from build123d import *

# Parameters (mm, degrees)
BASE_FLANGE1_DEPTH = 280
SKETCH2_W          = 105.722877612
SKETCH2_H          = 35.527417617
CUT_EXTRUDE1_DEPTH = 10
SKETCH3_R          = 38
CUT_EXTRUDE2_DEPTH = 500


# Sheet-metal steps are written as plain solids
with BuildPart() as part:
    # Sketch1 → Base-Flange1 (new body)
    with BuildSketch(Plane(origin=(0, 0, 0), x_dir=(-1, 0, 0), z_dir=(0, 0, 1))):
        with BuildLine():
            Line((223.448991217, -255.847131966), (223.448991217, 313.416268034))
            ThreePointArc((223.448991217, 313.416268034), (223.233246072, 313.937122889), (222.712391217, 314.152868034))
            Line((222.712391217, 314.152868034), (-112.814408783, 314.152868034))
            ThreePointArc((-112.814408783, 314.152868034), (-113.335263638, 313.937122889), (-113.551008783, 313.416268034))
            Line((-113.551008783, 313.416268034), (-113.551008783, -255.847131966))
            Line((-113.551008783, -255.847131966), (-115.051008783, -255.847131966))
            Line((-115.051008783, -255.847131966), (-115.051008783, 313.416268034))
            ThreePointArc((-115.051008783, 313.416268034), (-114.39592381, 314.997783061), (-112.814408783, 315.652868034))
            Line((-112.814408783, 315.652868034), (222.712391217, 315.652868034))
            ThreePointArc((222.712391217, 315.652868034), (224.293906243, 314.997783061), (224.948991217, 313.416268034))
            Line((224.948991217, 313.416268034), (224.948991217, -255.847131966))
            Line((224.948991217, -255.847131966), (223.448991217, -255.847131966))
        make_face()
    extrude(amount=BASE_FLANGE1_DEPTH)

    # Sketch2 → Cut-Extrude1 (cut)
    with BuildSketch(Plane.ZY.offset(224.948991217)):
        with Locations((233.67908011, -135.779600883)):
            Rectangle(SKETCH2_W, SKETCH2_H)
    extrude(amount=-CUT_EXTRUDE1_DEPTH, mode=Mode.SUBTRACT)

    # Sketch3 → Cut-Extrude2 (cut)
    with BuildSketch(Plane(origin=(0, -314.152868034, 0), x_dir=(1, 0, 0), z_dir=(0, 1, 0))):
        with Locations(Location((33.054236524, -81.51765287, 0), (0, 0, 180))):
            Circle(SKETCH3_R)
    extrude(amount=-CUT_EXTRUDE2_DEPTH, mode=Mode.SUBTRACT)


solid = part.part
Design review of the part built by this model. Coordinates are the model's own, in mm. A direction names the side the tool comes from. Round coordinates to 2 decimals unless told otherwise and drop trailing zeros. Write each loop counter-clockwise with the first axis right and the second up, starting at its lowest first coordinate (ties: lowest second). Pieces come first, ordered by that corner, then holes. Notation, with made-up numbers: (88, 64) - (139, 64) arc R19 cw to (139, 69) - close; hole circle Ø1 at (-27.75, -30.75). An arc over 180 degrees is marked (long way). Use a Markdown table: item, result. Add a question column.
1. We need section B-B (z = 203). State the section outline as (x, y) points.
2. We need section D-D (z = 168.5). State the section outline as (x, y) points.
3. Clearance check with flat-ended pins moving along their axes: pin 1 (1.2 mm diameter, centred on x = -224, y = -130.5, fed in from +Z); pin 2 (6 mm diameter, centred on x = -70.5, z = 67, fed in from +Y). State where each tip first meets the part, or that it passes through.
4. Wall thickness on probe 1 along X at (y, z) = (93, 173); probe 2 along Y at (x, z) = (46, 199.5); probe 3 along X at (y, z) = (-136, 240): over which ranges is each line inside the solid? List them lowest first.
5. We need section A-A (y = 93). State the section outline as (x, z) points.
6. We need section C-C (x = 30). State the section outline as (y, z) points.
7. For faces 5 (the face through (38.001, -314.892, 119.194)), 6 (the face through (113.551, -33, 138)), list the 3-axis set-ups (+Z, -Z, +X, -X, +Y, -Y) from which the entire face can be reached by the end or side of a thin tool; tool diameter is ignored.
8. Mouldability with a two-part tool opening along X and no side actions: class faces 1 (the face through (-53, -315.653, 138)), 2 (the face through (-223.449, -25, 138)), 3 (the face through (-57, -314.153, 138)), 4 (the face through (115.051, -25, 138)) as +X half, -X half, draft (parallel to the pull), parting line (faces both ways), or undercut.
Output:
| question | item | result |
|---|---|---|
| 1 | outline | (-224.95, -313.42) arc R2.24 ccw to (-222.71, -315.65) - (112.81, -315.65) arc R2.24 ccw to (115.05, -313.42) - (115.05, 255.85) - (113.55, 255.85) - (113.55, -313.42) arc R0.74 cw to (112.81, -314.15) - (-222.71, -314.15) arc R0.74 cw to (-223.45, -313.42) - (-223.45, -153.54) - (-224.95, -153.54) - close; (-224.95, -118.02) - (-223.45, -118.02) - (-223.45, 255.85) - (-224.95, 255.85) - close |
| 2 | outline | (-224.95, -313.42) arc R2.24 ccw to (-222.71, -315.65) - (112.81, -315.65) arc R2.24 ccw to (115.05, -313.42) - (115.05, 255.85) - (113.55, 255.85) - (113.55, -313.42) arc R0.74 cw to (112.81, -314.15) - (-222.71, -314.15) arc R0.74 cw to (-223.45, -313.42) - (-223.45, 255.85) - (-224.95, 255.85) - close |
| 3 | pin 1 | stops at z = 180.82 |
| 3 | pin 2 | stops at y = -314.15 |
| 4 | probe 1 | x = -224.95 to -223.45, 113.55 to 115.05 |
| 4 | probe 2 | y = -315.65 to -314.15 |
| 4 | probe 3 | x = 113.55 to 115.05 |
| 5 | outline | (-224.95, 0) - (-223.45, 0) - (-223.45, 280) - (-224.95, 280) - close; (113.55, 0) - (115.05, 0) - (115.05, 280) - (113.55, 280) - close |
| 6 | outline | (-315.65, 0) - (-314.15, 0) - (-314.15, 43.64) - (-315.65, 43.64) - close; (-315.65, 119.39) - (-314.15, 119.39) - (-314.15, 280) - (-315.65, 280) - close |
| 7 | face 5 | +Y, -Y |
| 7 | face 6 | +Z, -Z, +Y |
| 8 | face 1 | draft |
| 8 | face 2 | undercut |
| 8 | face 3 | undercut |
| 8 | face 4 | +X half |
